Source: CAD feature listing. Evaluate the final solid. Frame: model axes, mm. Face numbers are marked on the shaded views. Coordinates: 2 decimals unless noted, no trailing zeros. Order: outer loops, then holes, each group sorted by start corner. A loop starts at its lowest first (then second) coordinate and runs counter-clockwise, first axis right, second up. Notation, with made-up numbers: (46, -6.5) - (60, -6.5) arc R12 cw to (60, 15.5) - close; hole circle Ø10 at (50, 47.5). An arc over 180 degrees is marked (long way). One line per question, with ' | ' between items. Start each with the question number.
(1) Section B-B (z = 1.9). Return the cut outline in (x, y), then the cut area to 3 significant figures.
(2) Section A-A (x = 0). Return the cut outline in (y, z).
(3) Line query: line 1 along Y through (x, z) = (0, 2.7); line 2 along Y through (x, z) = (-1.5, 3.7); line 3 along X through (y, z) = (1.5, 0.55). Output: solid intervals per line, ascending.
(4) Contact query for flat-ended pins moving along their axis: P1, Ø1.5, axis at y = -12, z = 4, coming from the -X side; P2, Ø5, axis at x = 0, y = 0, coming from the -Z side; P3, Ø1.5, axis at y = -4.5, z = 5, coming from the +X side; P4, Ø1.5, axis at x = 15.5, y = -29.5, coming from the -Z side. Output: stop coordinate, or through.
(5) Draft query along X for the marked faces 1, 2 and 3. Return one class per face: +X half, -X half, draft (parallel to the pull), parting line (faces both ways), or undercut.
from build123d import *

# Parameters (mm, degrees)
F0_R     = 20
F0_R_2   = 2
F1_DEPTH = 6
F2_R     = 1


with BuildPart() as f1:
    # F0 (on Top) → F1 (new body)
    with BuildSketch(Plane.XY):
        with Locations((0, -15)):
            Circle(F0_R)
        Circle(F0_R_2, mode=Mode.SUBTRACT)
    extrude(amount=F1_DEPTH)

    # F2
    f2_edges = [f1.edges().sort_by_distance(p)[0] for p in [
        (-20, -15, 6),
        (-2, 0, 6),
        (-20, -15, 0),
        (-2, 0, 0),
    ]]
    fillet(f2_edges, radius=F2_R)


solid = f1.part
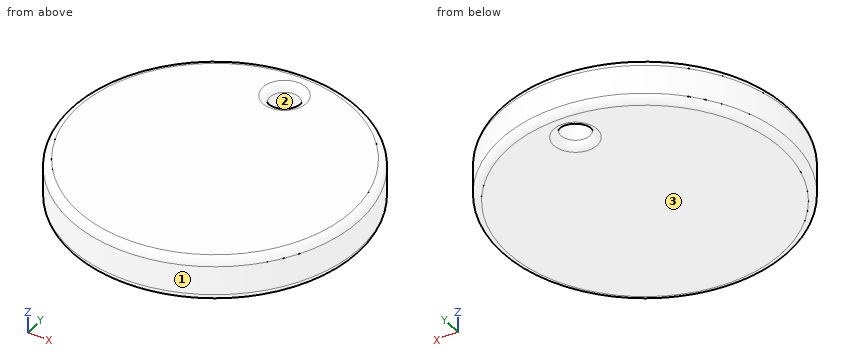
Response values:
1) outline: circle Ø40 at (0, -15); hole circle Ø4 at (0, 0) | area: 1,240 mm²
2) outline: (-35, 1) arc R1 ccw to (-34, 0) - (-3, 0) arc R1 ccw to (-2, 1) - (-2, 5) arc R1 ccw to (-3, 6) - (-34, 6) arc R1 ccw to (-35, 5) - close; (2, 1) arc R1 ccw to (3, 0) - (4, 0) arc R1 ccw to (5, 1) - (5, 5) arc R1 ccw to (4, 6) - (3, 6) arc R1 ccw to (2, 5) - close
3) line 1: y = -35 to -2, 2 to 5 | line 2: y = -34.94 to -1.32, 1.32 to 4.94 | line 3: x = -11.11 to -1.48, 1.48 to 11.11
4) P1: stops at x = -19.87 | P2: stops at z = 0.13 | P3: stops at x = 17.46 | P4: passes through
5) face 1: parting line | face 2: undercut | face 3: draft
